Check sheet for the modelled part. Datum: model origin and axes. Units: mm. A direction names the side the tool comes from. Round coordinates to 2 decimals unless told otherwise and drop trailing zeros. Loops run counter-clockwise (first coordinate to the right, second up) from the corner with the lowest first, then second, coordinate; pieces in that order, holes last. Notation, with made-up numbers: (57.5, 48) -> (92.5, 48) arc R10 ccw to (92.5, 63) -> close; hole circle Ø6 at (4, 46). An arc over 180 degrees is marked (long way). Return JSON: item names as keys, results as strings.
from build123d import *

# Parameters (mm, degrees)
BOSS_EXTRUDE1_DEPTH = 5
SKETCH2_R           = 2.5
CUT_EXTRUDE1_DEPTH  = 74.739406019
BOSS_EXTRUDE3_START = 5
SKETCH7_R           = 9
BOSS_EXTRUDE3_DEPTH = 5
SKETCH8_R           = 5.5
CUT_EXTRUDE3_DEPTH  = 75.246212025
SKETCH9_R           = 1.55
CUT_EXTRUDE4_DEPTH  = 74.739406019


with BuildPart() as part:
    # Sketch1 → Boss-Extrude1 (new body)
    with BuildSketch(Plane(origin=(0, 0, 0), x_dir=(1, 0, 0), z_dir=(0, 1, 0))):
        with BuildLine():
            Line((0, 9), (51.325324214, 9))
            ThreePointArc((51.325324214, 9), (72.5, 0), (51.325324214, -9))
            Line((51.325324214, -9), (0, -9))
            ThreePointArc((0, -9), (-9, 0), (0, 9))
        make_face()
    extrude(amount=BOSS_EXTRUDE1_DEPTH)

    # Sketch2 → Cut-Extrude1 (cut, through all)
    with BuildSketch(Plane(origin=(0, 5, 0), x_dir=(1, 0, 0), z_dir=(0, 1, 0))):
        with Locations(Location((60, 0, 0), (0, 0, 270))):
            Circle(SKETCH2_R)
    extrude(amount=-CUT_EXTRUDE1_DEPTH, mode=Mode.SUBTRACT)

    # Sketch7 → Boss-Extrude3 (add)
    with BuildSketch(Plane.XZ.offset(BOSS_EXTRUDE3_START)):
        with Locations(Location((0, 0, 0), (0, 0, 270))):
            Circle(SKETCH7_R)
    extrude(amount=-BOSS_EXTRUDE3_DEPTH)

    # Sketch8 → Cut-Extrude3 (cut, through all)
    with BuildSketch(Plane.XZ.offset(5)):
        with Locations(Location((0, 0, 0), (0, 0, 270))):
            Circle(SKETCH8_R)
    extrude(amount=-CUT_EXTRUDE3_DEPTH, mode=Mode.SUBTRACT)

    # Sketch9 → Cut-Extrude4 (cut, through all)
    with BuildSketch(Plane.XZ):
        with Locations(Location((60, 8, 0), (0, 0, 270))):
            Circle(SKETCH9_R)
        with Locations(Location((60, -8, 0), (0, 0, 270))):
            Circle(SKETCH9_R)
        with Locations(Location((68, 0, 0), (0, 0, 270))):
            Circle(SKETCH9_R)
        with Locations(Location((52, 0, 0), (0, 0, 270))):
            Circle(SKETCH9_R)
    extrude(amount=-CUT_EXTRUDE4_DEPTH, mode=Mode.SUBTRACT)


solid = part.part
Q1. Section check C-C (y = 1.75). Record the boundary of the cut face in (x, z).
Results list:
{"outline": "(0, -9) -> (51.33, -9) arc R12.5 ccw (long way) to (51.33, 9) -> (0, 9) arc R9 ccw to start; hole circle Ø11 at (0, 0); hole circle Ø3.1 at (52, 0); hole circle Ø5 at (60, 0); hole circle Ø3.1 at (60, -8); hole circle Ø3.1 at (60, 8); hole circle Ø3.1 at (68, 0)"}
Q2. Tool access check on faces 1 (the flat face through (25, 2, -9)), 2 (the flat face through (26, 2, 9)), 3 (the cylindrical face through (-5.37, -0.07, 1.19)). Record the directions out of +Z, -Z, +X, -X, +Y, -Y that give a thin tool (end or side, any length) a straight path to the whole face; none if there is none.
Results list:
{"face 1": "-Z, -X, +Y, -Y", "face 2": "+Z, -X, +Y, -Y", "face 3": "+Y, -Y"}
Q3. Draft check along Z on faces 4 (the cylindrical face through (72.493, 2.465, -0.409)), 5 (the cylindrical face through (57.56, 2.54, -0.54)), 6 (the flat face through (-4, -5, 4)). Enter one of: released by +Z, released by -Z, zero draft, split by the parting line, or undercut.
Results list:
{"face 4": "split by the parting line", "face 5": "undercut", "face 6": "zero draft"}
Q4. Section check B-B (z = 0). Record the boundary of the cut face in (x, y), then the cut area to 4 significant figures.
Results list:
{"outline": "(-9, -5) -> (-5.5, -5) -> (-5.5, 5) -> (-9, 5) -> close; (5.5, -5) -> (9, -5) -> (9, 0) -> (50.45, 0) -> (50.45, 5) -> (5.5, 5) -> close; (53.55, 0) -> (57.5, 0) -> (57.5, 5) -> (53.55, 5) -> close; (62.5, 0) -> (66.45, 0) -> (66.45, 5) -> (62.5, 5) -> close; (69.55, 0) -> (72.5, 0) -> (72.5, 5) -> (69.55, 5) -> close", "area": "331.5 mm^2"}
Q5. Material ranges on line 1 (X direction, y = 1.5, z = -1.75); line 2 (X direction, y = 1.75, z = -0.5); line 3 (Y direction, x = 48.5, z = 2.5), recorded low to high.
Results list:
{"line 1": "-8.83 to -5.21, 5.21 to 58.21, 61.79 to 72.38", "line 2": "-8.99 to -5.48, 5.48 to 50.53, 53.47 to 57.55, 62.45 to 66.53, 69.47 to 72.49", "line 3": "0 to 5"}
Q6. Go/stop test with flat-tipped pins: pin 1 (4 mm diameter, centred on x = 39.5, z = -1.5, fed in from -Y); pin 2 (1.5 mm diameter, centred on y = 3, z = -3.5, fed in from -X); pin 3 (5 mm diameter, centred on x = 25.5, y = 1.5, fed in from -Z). Record where each tip stops, or that it passes through.
Results list:
{"pin 1": "y = 0", "pin 2": "x = -8.57", "pin 3": "z = -9"}
Q7. Section check A-A (x = 60). Record the boundary of the cut face in (y, z).
Results list:
{"outline": "(0, -12.5) -> (5, -12.5) -> (5, -9.55) -> (0, -9.55) -> close; (0, -6.45) -> (5, -6.45) -> (5, -2.5) -> (0, -2.5) -> close; (0, 2.5) -> (5, 2.5) -> (5, 6.45) -> (0, 6.45) -> close; (0, 9.55) -> (5, 9.55) -> (5, 12.5) -> (0, 12.5) -> close"}
Q8. Section check D-D (z = 3.75). Record the boundary of the cut face in (x, y), then the cut area to 3 significant figures.
Results list:
{"outline": "(-8.18, -5) -> (-4.02, -5) -> (-4.02, 5) -> (-8.18, 5) -> close; (4.02, -5) -> (8.18, -5) -> (8.18, 0) -> (71.92, 0) -> (71.92, 5) -> (4.02, 5) -> close", "area": "402 mm^2"}
